Autodesk Inventor part; units mm, degrees
ref_plane "YZ Plane" through (0, 0, 0) normal (1, 0, 0) x (0, 1, 0)
ref_plane "XZ Plane" through (0, 0, 0) normal (0, 1, 0) x (-1, 0, 0)
ref_plane "XY Plane" through (0, 0, 0) normal (0, 0, 1) x (1, 0, 0)
sketch "Sketch1" plane through (0, 0, 0) normal (0, 1, 0) x (-1, 0, 0)
  line L0 (0, 0) -> (-190.5, 0)
  line L1 (-190.5, 0) -> (-190.5, -190.5)
  line L2 (-190.5, -190.5) -> (0, -190.5)
  line L3 (0, -190.5) -> (0, 0)
  circle A0 centre (-79.375, -79.375) radius 47.625
  line L4 (-25.4, -190.5) -> (-25.4, 0) construction
  line L5 (0, -25.4) -> (-190.5, -25.4) construction
  line L6 (0, 0) -> (-190.5, -190.5) construction
  circle A1 centre (-79.375, -79.375) radius 53.975 construction
  dimension "d0" = 95.25
  dimension "d3" = 25.4
  dimension "d4" = 25.4
  dimension "d5" = 107.95
  dimension "d48" = 165.1
extrude "Extrusion1" add sketch "Sketch1" along normal blind 6.35
sketch "Sketch2" plane through (0, 6.35, 0) normal (0, 1, 0) x (1, 0, 0)
  circle A0 centre (79.375, 79.375) radius 47.625 construction
  circle A1 centre (79.375, 79.375) radius 57.15 construction
  line L0 (0, 190.5) -> (0, 0) construction
  arc A2 (177.8, 76.2) -> (76.2, 177.8) centre (76.2, 76.2) ccw construction
  line L1 (38.9638, 38.9638) -> (119.7862, 38.9638) construction
  line L2 (119.7862, 38.9638) -> (119.7862, 119.7862) construction
  line L3 (119.7862, 119.7862) -> (38.9638, 119.7862) construction
  line L4 (38.9638, 119.7862) -> (38.9638, 38.9638) construction
  dimension "d9" = 114.3
hole "Hole1" at (38.9638, 6.35, -38.9638) at (119.7862, 6.35, -119.7862) at (119.7862, 6.35, -38.9638) at (38.9638, 6.35, -119.7862) direction (0, -1, 0) diameter 4.9784 end through all
sketch "Sketch4" plane through (0, 6.35, 0) normal (0, 1, 0) x (1, 0, 0)
  line L0 (0, 0) -> (190.5, 0)
  line L1 (0, 0) -> (25.4, 0)
  line L2 (25.4, 0) -> (25.4, 69.85)
  line L3 (25.4, 69.85) -> (0, 69.85)
  line L4 (0, 69.85) -> (0, 0)
  line L5 (25.4, 0) -> (69.85, 0)
  line L6 (69.85, 0) -> (69.85, 25.4)
  line L7 (69.85, 25.4) -> (25.4, 25.4)
  line L8 (25.4, 25.4) -> (25.4, 0)
  dimension "d26" = 25.4
  dimension "d27" = 69.85
  dimension "d28" = 44.45
  dimension "d29" = 25.4
extrude "Extrusion3" cut sketch "Sketch4" against normal through all
sketch "Sketch5" plane through (0, 6.35, 0) normal (0, 1, 0) x (1, 0, 0)
  circle A0 centre (154.1438, 85.8655) radius 11.1125
  circle A1 centre (79.375, 79.375) radius 47.625 construction
  circle A2 centre (79.375, 79.375) radius 75.05 construction
  circle A3 centre (153.2048, 55.4) radius 25.4 construction
  circle A4 centre (119.7862, 38.9638) radius 2.4892 construction
  circle A5 centre (38.9638, 38.9638) radius 2.4892 construction
  circle A6 centre (119.7862, 119.7862) radius 2.4892 construction
  line L0 (38.9638, 38.9638) -> (119.7862, 119.7862) construction
  circle A7 centre (85.8655, 154.1438) radius 11.1125
  circle A8 centre (153.2048, 55.4) radius 7.62 construction
  circle A9 centre (154.1438, 85.8655) radius 22.86 construction
  line L1 (69.85, 0) -> (69.85, 25.4) construction
  line L2 (69.85, 25.4) -> (168.2375, 25.4) construction
  circle A10 centre (153.2048, 55.4) radius 30 construction
  circle A11 centre (153.2048, 55.4) radius 9.525
  circle A12 centre (55.4, 153.2048) radius 9.525
  circle A13 centre (79.375, 79.375) radius 47.625
  point P0 (0, 0)
  dimension "d38" = 150.1
  dimension "d37" = 22.225
  dimension "d43" = 15.24
  dimension "d44" = 45.72
  dimension "d46" = 50.8
  dimension "d47" = 60
  dimension "d72" = 19.05
extrude "Extrusion4" cut sketch "Sketch5" against normal through all contours A0 | A7
sketch "Sketch6" plane through (0, 6.35, 0) normal (0, 1, 0) x (1, 0, 0)
  line L0 (69.85, 0) -> (190.5, 0)
  line L1 (0, 190.5) -> (0, 69.85)
  point P0 (0, 0)
  point P1 (12.7, 12.7)
  point P2 (76.2, 0)
  point P3 (184.15, 0)
  point P4 (25.4, 12.7)
  point P5 (38.1, 12.7)
  point P6 (50.8, 12.7)
  point P7 (63.5, 12.7)
  point P8 (76.2, 12.7)
  point P9 (88.9, 12.7)
  point P10 (101.6, 12.7)
  point P11 (114.3, 12.7)
  point P12 (127, 12.7)
  point P13 (139.7, 12.7)
  point P14 (152.4, 12.7)
  point P15 (165.1, 12.7)
  point P16 (177.8, 12.7)
  point P17 (0, 184.15)
  point P18 (0, 76.2)
  point P19 (12.7, 25.4)
  point P20 (12.7, 38.1)
  point P21 (12.7, 50.8)
  point P22 (12.7, 63.5)
  point P23 (12.7, 76.2)
  point P24 (12.7, 88.9)
  point P25 (12.7, 101.6)
  point P26 (12.7, 114.3)
  point P27 (12.7, 127)
  point P28 (12.7, 139.7)
  point P29 (12.7, 152.4)
  point P30 (12.7, 165.1)
  point P31 (12.7, 177.8)
  dimension "d49" = 12.7
  dimension "d50" = 12.7
  dimension "d53" = 12.7
  dimension "d60" = 12.7
hole "Hole2" at (12.7, 6.35, -12.7) at (25.4, 6.35, -12.7) at (38.1, 6.35, -12.7) at (50.8, 6.35, -12.7) at (63.5, 6.35, -12.7) at (76.2, 6.35, -12.7) at (88.9, 6.35, -12.7) at (101.6, 6.35, -12.7) at (114.3, 6.35, -12.7) at (127, 6.35, -12.7) at (139.7, 6.35, -12.7) at (152.4, 6.35, -12.7) at (165.1, 6.35, -12.7) at (177.8, 6.35, -12.7) at (12.7, 6.35, -25.4) at (12.7, 6.35, -38.1) at (12.7, 6.35, -50.8) at (12.7, 6.35, -63.5) at (12.7, 6.35, -76.2) at (12.7, 6.35, -88.9) at (12.7, 6.35, -101.6) at (12.7, 6.35, -114.3) at (12.7, 6.35, -127) at (12.7, 6.35, -139.7) at (12.7, 6.35, -152.4) at (12.7, 6.35, -165.1) at (12.7, 6.35, -177.8) direction (0, -1, 0) diameter 4.9784 end through all
sketch "Sketch8" plane through (0, 6.35, 0) normal (0, 1, 0) x (1, 0, 0)
  circle A0 centre (85.8655, 154.1438) radius 11.1125
  circle A1 centre (85.8655, 154.1438) radius 17.4625
  circle A2 centre (154.1438, 85.8655) radius 11.1125
  circle A3 centre (154.1438, 85.8655) radius 17.4625
  line L0 (85.8655, 171.6063) -> (0, 171.6063)
  line L1 (0, 190.5) -> (0, 69.85)
  line L2 (171.6063, 85.8655) -> (171.6063, 0)
  line L3 (69.85, 0) -> (190.5, 0)
  line L4 (98.2134, 166.4917) -> (166.4917, 98.2134)
  line L5 (190.5, 190.5) -> (0, 190.5)
  line L6 (190.5, 0) -> (190.5, 190.5)
  line L7 (28.575, 165.2563) -> (66.8155, 165.2563)
  arc A4 (69.7463, 160.8602) -> (76.9719, 139.1158) centre (85.8655, 154.1438) ccw
  circle A5 centre (79.375, 79.375) radius 47.625
  circle A6 centre (38.9638, 119.7862) radius 2.4892
  arc A7 (75.5782, 133.2163) -> (48.1037, 123.3683) centre (79.375, 79.375) ccw
  arc A8 (35.3817, 110.6463) -> (31.3972, 104.1022) centre (79.375, 79.375) ccw
  arc A9 (25.4, 105.5567) -> (31.3972, 104.1022) centre (28.575, 105.5567) ccw
  arc A10 (28.575, 165.2563) -> (25.4, 162.0813) centre (28.575, 162.0813) ccw
  arc A11 (69.7463, 160.8602) -> (66.8155, 165.2563) centre (66.8155, 162.0813) ccw
  arc A12 (75.5782, 133.2163) -> (76.9719, 139.1158) centre (75.3548, 136.3834) ccw
  arc A13 (44.0192, 123.7111) -> (48.1037, 123.3683) centre (46.2643, 125.9561) ccw
  arc A14 (35.3817, 110.6463) -> (35.0389, 114.7308) centre (32.7939, 112.4857) ccw
  line L8 (25.4, 69.85) -> (25.4, 25.4)
  line L9 (107.1936, 148.5312) -> (121.1272, 134.5976)
  line L10 (121.1272, 130.1075) -> (114.7308, 123.7111)
  arc A15 (110.6463, 123.3683) -> (92.3928, 131.7566) centre (79.375, 79.375) ccw
  arc A16 (92.0366, 137.8081) -> (102.0127, 147.495) centre (85.8655, 154.1438) ccw
  circle A17 centre (119.7862, 119.7862) radius 2.4892 construction
  line L11 (79.375, 79.375) -> (119.7862, 119.7862) construction
  arc A18 (92.0366, 137.8081) -> (92.3928, 131.7566) centre (93.1586, 134.8379) ccw
  arc A19 (107.1936, 148.5312) -> (102.0127, 147.495) centre (104.9486, 146.2861) ccw
  arc A20 (121.1272, 130.1075) -> (121.1272, 134.5976) centre (118.8821, 132.3525) ccw
  arc A21 (110.6463, 123.3683) -> (114.7308, 123.7111) centre (112.4857, 125.9561) ccw
  line L12 (148.5312, 107.1936) -> (134.5976, 121.1272)
  line L13 (130.1075, 121.1272) -> (123.7111, 114.7308)
  arc A22 (131.7566, 92.3928) -> (123.3683, 110.6463) centre (79.375, 79.375) ccw
  arc A23 (147.495, 102.0127) -> (137.8081, 92.0366) centre (154.1438, 85.8655) ccw
  arc A24 (131.7566, 92.3928) -> (137.8081, 92.0366) centre (134.8379, 93.1586) ccw
  arc A25 (147.495, 102.0127) -> (148.5312, 107.1936) centre (146.2861, 104.9486) ccw
  arc A26 (134.5976, 121.1272) -> (130.1075, 121.1272) centre (132.3525, 118.8821) ccw
  arc A27 (123.7111, 114.7308) -> (123.3683, 110.6463) centre (125.9561, 112.4857) ccw
  line L14 (35.0389, 114.7308) -> (30.8201, 118.9497)
  line L15 (44.0192, 123.7111) -> (26.3299, 141.4003)
  line L16 (79.375, 79.375) -> (38.9638, 119.7862) construction
  line L17 (25.4, 162.0813) -> (25.4, 143.6454)
  line L18 (25.4, 116.7046) -> (25.4, 105.5567)
  arc A28 (25.4, 143.6454) -> (26.3299, 141.4003) centre (28.575, 143.6454) ccw
  arc A29 (30.8201, 118.9497) -> (25.4, 116.7046) centre (28.575, 116.7046) ccw
  line L19 (165.2563, 28.575) -> (165.2563, 66.8155)
  arc A30 (139.1158, 76.9719) -> (160.8602, 69.7463) centre (154.1438, 85.8655) ccw
  arc A31 (123.3683, 48.1037) -> (133.2163, 75.5782) centre (79.375, 79.375) ccw
  arc A32 (104.1022, 31.3972) -> (110.6463, 35.3817) centre (79.375, 79.375) ccw
  arc A33 (104.1022, 31.3972) -> (105.5567, 25.4) centre (105.5567, 28.575) ccw
  arc A34 (162.0813, 25.4) -> (165.2563, 28.575) centre (162.0813, 28.575) ccw
  arc A35 (165.2563, 66.8155) -> (160.8602, 69.7463) centre (162.0813, 66.8155) ccw
  arc A36 (139.1158, 76.9719) -> (133.2163, 75.5782) centre (136.3834, 75.3548) ccw
  arc A37 (123.3683, 48.1037) -> (123.7111, 44.0192) centre (125.9561, 46.2643) ccw
  arc A38 (114.7308, 35.0389) -> (110.6463, 35.3817) centre (112.4857, 32.7939) ccw
  line L20 (114.7308, 35.0389) -> (118.9497, 30.8201)
  line L21 (123.7111, 44.0192) -> (141.4003, 26.3299)
  line L22 (162.0813, 25.4) -> (143.6454, 25.4)
  line L23 (116.7046, 25.4) -> (105.5567, 25.4)
  arc A39 (141.4003, 26.3299) -> (143.6454, 25.4) centre (143.6454, 28.575) ccw
  arc A40 (116.7046, 25.4) -> (118.9497, 30.8201) centre (116.7046, 28.575) ccw
  point P0 (0, 0)
  point P1 (160.8602, 69.7463)
  point P2 (139.1158, 76.9719)
  dimension "d94" = 34.925
  dimension "d98" = 3.175
  dimension "d99" = 6.35
  dimension "d102" = 6.35
  dimension "d103" = 6.35
  dimension "d105" = 6.35
  dimension "d108" = 6.35
  dimension "d109" = 6.35
  dimension "d113" = 6.35
  dimension "d114" = 6.35
extrude "Extrusion6" cut sketch "Sketch8" against normal through all contours A1 L0 L1 L5 L6 L3 L2 A3 L4 | A19 L9 A20 L10 A21 A15 A18 A1 | A1 A12 A7 A13 L15 A28 L17 A10 L7 A11 | A3 A24 A22 A27 L13 A26 L12 A25 | A35 L19 A34 L22 A39 L21 A37 A31 A36 A3 | A8 A9 L18 A29 L14 A14 | A32 A38 L20 A40 L23 A33
fillet "Fillet7" radius 6.35 5 edges at (25.4, 3.175, -25.4) (69.85, 3.175, 0) (171.6063, 3.175, 0) (0, 3.175, -69.85) (0, 3.175, -171.6063)
properties part number "Plate_Bottom" material "Aluminum 6061"
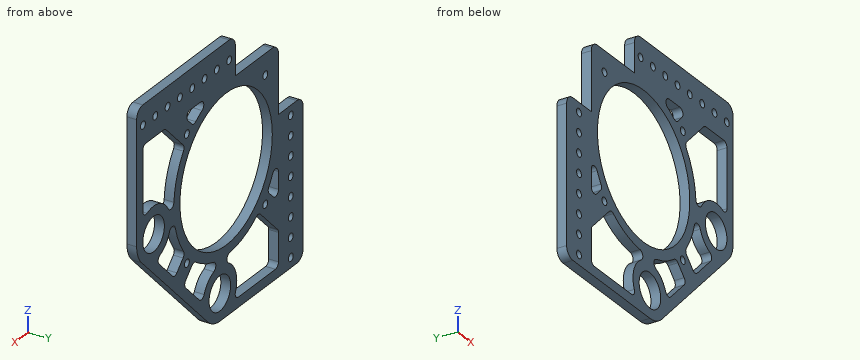
Verification items for the finished model (mm, model axes). Give positions to 0.01 mm unless a question says otherwise; leave off trailing zeros. Order: outer loops, then holes, each group sorted by start corner. A loop starts at its lowest first (then second) coordinate and runs counter-clockwise, first axis right, second up. Notation, with made-up numbers: (-8, 18.5) -> (38, 18.5) arc R29 ccw to (38, 51.5) -> close; hole circle Ø8 at (20, 38.5). An arc over 180 degrees is marked (long way). Use a Markdown table: item, result.
1) Material ranges on probe 1 along Z at (x, y) = (41.5, 6); probe 2 along Z at (x, y) = (62, 2); probe 3 along X at (y, z) = (5.5, -77.5), recorded low to high.
Results:
| item | result |
|---|---|
| probe 1 | -171.61 to -165.26, -126.23 to -108.25, -50.5 to -25.4 |
| probe 2 | -171.61 to -165.26, -130.48 to -123.72, -35.03 to -25.4 |
| probe 3 | 0 to 10.58, 14.82 to 31.79, 126.96 to 134.04, 138.72 to 146.83, 161.46 to 171.61 |
2) Section check B-B, the plane y = 3.75. Give the number of separate pieces and of enclosed holes in the cut face, then the cut area to 3 significant figures.
Results:
| item | result |
|---|---|
| separate pieces | 1 |
| enclosed holes | 29 |
| area | 10,700 mm² |
3) Depth check by flat-ended pin: pin 1 Ø5.5 at (x, z) = (119.79, -119.79) entering from -Y; pin 2 Ø1.9 at (x, y) = (111.5, 4.5) entering from -Z; pin 3 Ø3 at (y, z) = (4.5, -56.5) entering from -X; pin 4 Ø1.5 at (y, z) = (3, -108.5) entering from +X. Enter the tip coordinate at first touch or a pass-through.
Results:
| item | result |
|---|---|
| pin 1 | y = 0 |
| pin 2 | z = -154.16 |
| pin 3 | x = 25.4 |
| pin 4 | x = 156.96 |
4) Section check A-A, the plane x = 56.5. Record the boundary of the cut face in (y, z).
Results:
| item | result |
|---|---|
| outline | (0, -171.61) -> (6.35, -171.61) -> (6.35, -165.26) -> (0, -165.26) -> close; (0, -128.26) -> (6.35, -128.26) -> (6.35, -121.15) -> (0, -121.15) -> close; (0, -37.6) -> (6.35, -37.6) -> (6.35, -25.4) -> (0, -25.4) -> close |
5) Section check C-C, the plane x = 22.5. Record the boundary of the cut face in (y, z), then the cut area to 3 significant figures.
Results:
| item | result |
|---|---|
| outline | (0, -171.61) -> (6.35, -171.61) -> (6.35, -69.85) -> (0, -69.85) -> close |
| area | 646 mm² |
